Source: CAD feature listing. Evaluate the final solid. Frame: model axes, mm. Face numbers are marked on the shaded views. Give positions to 0.01 mm unless a question says otherwise; leave off trailing zeros. Write each loop counter-clockwise with the first axis right and the second up, starting at its lowest first coordinate (ties: lowest second). Pieces come first, ordered by that corner, then holes.
```python
from build123d import *

# Parameters (mm, degrees)
SKETCH2_W           = 22.225
SKETCH2_H           = 22.225
SKETCH2_W_2         = 13.97
SKETCH2_H_2         = 13.97
BOSS_EXTRUDE1_DEPTH = 6.35
SKETCH3_W           = 8.382
SKETCH3_H           = 3.81
CUT_EXTRUDE1_DEPTH  = 2.54
BOSS_EXTRUDE2_DEPTH = 8.382
SKETCH6_W           = 22.225
SKETCH6_H           = 22.225
SKETCH6_W_2         = 13.97
SKETCH6_H_2         = 13.97
BOSS_EXTRUDE3_DEPTH = 222.25
SKETCH7_W           = 22.225
SKETCH7_H           = 22.225
BOSS_EXTRUDE4_DEPTH = 6.35
SKETCH8_W           = 11.1125
SKETCH8_H           = 22.225
CUT_EXTRUDE2_DEPTH  = 33.02


with BuildPart() as part:
    # Sketch2 → Boss-Extrude1 (new body)
    with BuildSketch(Plane(origin=(0, 0, 0), x_dir=(1, 0, 0), z_dir=(0, 1, 0))):
        Rectangle(SKETCH2_W, SKETCH2_H)
        Rectangle(SKETCH2_W_2, SKETCH2_H_2, mode=Mode.SUBTRACT)
    extrude(amount=BOSS_EXTRUDE1_DEPTH)

    # Sketch3 → Cut-Extrude1 (cut)
    with BuildSketch(Plane(origin=(-6.985, 0, 0), x_dir=(0, 0, -1), z_dir=(1, 0, 0))):
        with Locations((0, 3.175)):
            Rectangle(SKETCH3_W, SKETCH3_H)
    extrude(amount=-CUT_EXTRUDE1_DEPTH, mode=Mode.SUBTRACT)

    # Sketch4 → Boss-Extrude2 (add)
    with BuildSketch(Plane(origin=(0, 0, 4.191), x_dir=(-1, 0, 0), z_dir=(0, 0, -1))):
        with BuildLine():
            Line((6.985, 4.191), (6.985, 2.159))
            ThreePointArc((6.985, 2.159), (8.001, 3.175), (6.985, 4.191))
        make_face()
    extrude(amount=BOSS_EXTRUDE2_DEPTH)

    # Sketch6 → Boss-Extrude3 (add)
    with BuildSketch(Plane(origin=(0, 6.35, 0), x_dir=(1, 0, 0), z_dir=(0, 1, 0))):
        Rectangle(SKETCH6_W, SKETCH6_H)
        Rectangle(SKETCH6_W_2, SKETCH6_H_2, mode=Mode.SUBTRACT)
    extrude(amount=BOSS_EXTRUDE3_DEPTH)

    # Sketch7 → Boss-Extrude4 (add)
    with BuildSketch(Plane(origin=(0, 228.6, 0), x_dir=(1, 0, 0), z_dir=(0, 1, 0))):
        Rectangle(SKETCH7_W, SKETCH7_H)
    extrude(amount=BOSS_EXTRUDE4_DEPTH)

    # Sketch8 → Cut-Extrude2 (cut)
    with BuildSketch(Plane.XZ):
        with Locations((5.55625, 0)):
            Rectangle(SKETCH8_W, SKETCH8_H)
    extrude(amount=-CUT_EXTRUDE2_DEPTH, mode=Mode.SUBTRACT)


solid = part.part
```
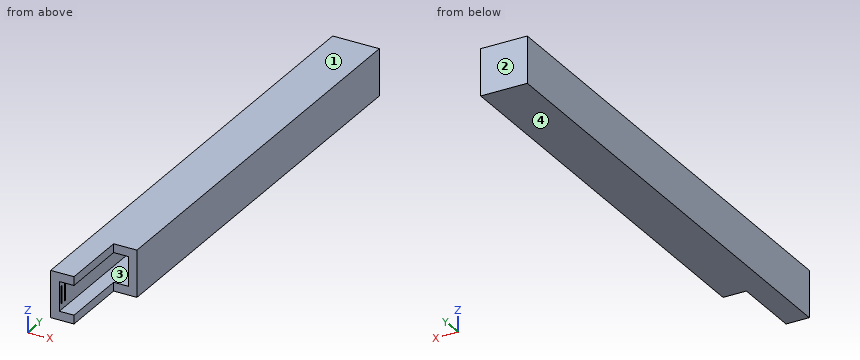
1. Section query B-B (y = 97). Return loops of the section in (x, z) (1 decimal).
2. Line query: probe 1 along X at (y, z) = (207, 2.75) (1 decimal); probe 2 along Y at (x, z) = (1.25, 8). Output: solid intervals per line, ascending.
3. Pull-direction query (Z, two-part tool) for the marked faces 1, 2, 3 and 4; classes: pulls with the +Z half, pulls with the -Z half, needs draft (parallel to the pull), parting line crosses it, or undercut.
4. Pin query (flat end, axial travel): P1, Ø4, axis at y = 2.5, z = 2, coming from the +X side (3 decimals); P2, Ø3.5, axis at y = 14, z = -9.5, coming from the +X side; P3, Ø9, axis at x = 6.5, z = 3.5, coming from the -Y side. Return the tip coordinate at first contact, or that it passes through.
The answers:
1. outline: (-11.1, -11.1) - (11.1, -11.1) - (11.1, 11.1) - (-11.1, 11.1) - close; hole (-7, -7) - (7, -7) - (7, 7) - (-7, 7) - close
2. probe 1: x = -11.1 to -7, 7 to 11.1
2. probe 2: y = 33.02 to 234.95
3. face 1: pulls with the +Z half
3. face 2: needs draft
3. face 3: undercut
3. face 4: pulls with the -Z half
4. P1: stops at x = -6.985
4. P2: stops at x = 0
4. P3: stops at y = 33.02
